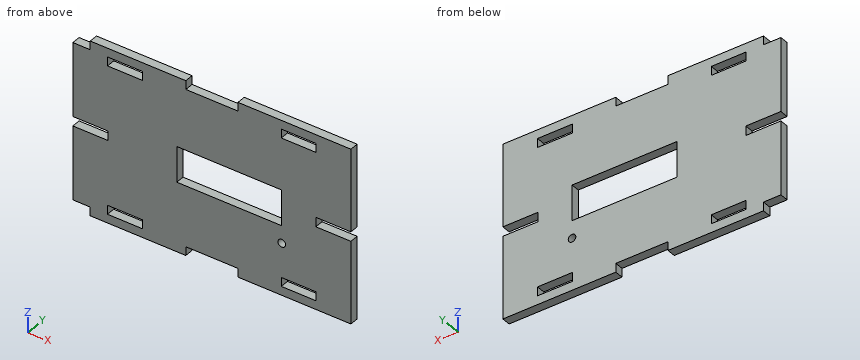
from build123d import *

# Parameters (mm, degrees)
SKETCH1_R           = 2.778125
SKETCH1_W           = 76.708
SKETCH1_H           = 25.908
BOSS_EXTRUDE1_DEPTH = 6.35
SKETCH4_W           = 12.7
SKETCH4_H           = 6.35
SKETCH4_W_2         = 25.5524
SKETCH4_H_2         = 6.5024
SKETCH4_W_3         = 38.1
CUT_EXTRUDE1_DEPTH  = 240.70724332


with BuildPart() as part:
    # Sketch1 → Boss-Extrude1 (new body)
    with BuildSketch(Plane(origin=(0, 0, 0), x_dir=(1, 0, 0), z_dir=(0, 1, 0))):
        Polygon((0, 0), (203.2, 0), (203.2, 60.071), (177.546, 60.071), (177.546, 66.929), (203.2, 66.929), (203.2, 127), (0, 127), (0, 66.929), (25.654, 66.929), (25.654, 60.071), (0, 60.071), align=None)
        with Locations(Location((152.654, 89.154, 0), (0, 0, 270))):
            Circle(SKETCH1_R, mode=Mode.SUBTRACT)
        with Locations((114.3, 63.5)):
            Rectangle(SKETCH1_W, SKETCH1_H, mode=Mode.SUBTRACT)
    extrude(amount=BOSS_EXTRUDE1_DEPTH)

    # Sketch4 → Cut-Extrude1 (cut, through all)
    with BuildSketch(Plane(origin=(0, 6.35, 0), x_dir=(1, 0, 0), z_dir=(0, 1, 0))):
        with Locations((6.35, 123.825)):
            Rectangle(SKETCH4_W, SKETCH4_H)
        with Locations((38.1, 117.3988)):
            Rectangle(SKETCH4_W_2, SKETCH4_H_2)
        with Locations((101.6, 123.825)):
            Rectangle(SKETCH4_W_3, SKETCH4_H)
        with Locations((165.1, 117.3988)):
            Rectangle(SKETCH4_W_2, SKETCH4_H_2)
        with Locations((165.1, 9.6012)):
            Rectangle(SKETCH4_W_2, SKETCH4_H_2)
        with Locations((101.6, 3.175)):
            Rectangle(SKETCH4_W_3, SKETCH4_H)
        with Locations((38.1, 9.6012)):
            Rectangle(SKETCH4_W_2, SKETCH4_H_2)
        with Locations((6.35, 3.175)):
            Rectangle(SKETCH4_W, SKETCH4_H)
    extrude(amount=-CUT_EXTRUDE1_DEPTH, mode=Mode.SUBTRACT)


solid = part.part
Can you work these out from the model? Positions are in its coordinate system, mm. Give positions to 0.01 mm unless a question says otherwise; leave off trailing zeros. Write each loop counter-clockwise with the first axis right and the second up, starting at its lowest first coordinate (ties: lowest second). Pieces come first, ordered by that corner, then holes. Notation, with made-up numbers: M 3,-16 L 58,-16 A20 ccw 58,15 Z; hole C -30,-7.5 d8. An arc over 180 degrees is marked long. Answer in a Markdown table with one row per item. Add a question column.
Item 1: For pin 1 Ø4.5 at (x, z) = (152.654, -89.154) entering from -Y, with a flat end and sliding along its axis, tell me the tip position at first contact or that it passes through.
Item 2: Imagine slicing it at B-B, the plane x = 20.5. Write out the boundary of the cut face in (y, z).
Item 3: Imagine slicing it at A-A, the plane x = 87.5. Write out the boundary of the cut face in (y, z).
Item 4: Imagine slicing it at C-C, the plane y = 2.5. State how many separate pieces and enclosed holes the cut face has, plus the area to 3 significant figures.
Item 5: Please list where these lines run through material, in increasing order: L1, parallel to Z at x = 173, y = 1.25; L2, parallel to Z at x = 136.5, y = 5.5; L3, parallel to X at y = 1.5, z = -115.
Evaluation:
| question | item | result |
|---|---|---|
| 1 | pin 1 | passes through |
| 2 | outline | M 0,-127 L 6.35,-127 L 6.35,-66.93 L 0,-66.93 Z; M 0,-60.07 L 6.35,-60.07 L 6.35,0 L 0,0 Z |
| 3 | outline | M 0,-120.65 L 6.35,-120.65 L 6.35,-76.45 L 0,-76.45 Z; M 0,-50.55 L 6.35,-50.55 L 6.35,-6.35 L 0,-6.35 Z |
| 4 | separate pieces | 1 |
| 4 | enclosed holes | 6 |
| 4 | area | 22,100 mm² |
| 5 | L1 | z = -127 to -120.65, -114.15 to -12.85, -6.35 to 0 |
| 5 | L2 | z = -127 to -76.45, -50.55 to 0 |
| 5 | L3 | x = 0 to 25.32, 50.88 to 152.32, 177.88 to 203.2 |
